Here's how the part is built. I have some questions about the finished solid (model axes, mm). Face numbers are marked on the shaded views. Coordinates: 2 decimals unless noted, no trailing zeros. Use one line per item in the form item = value. Start each with the question number.
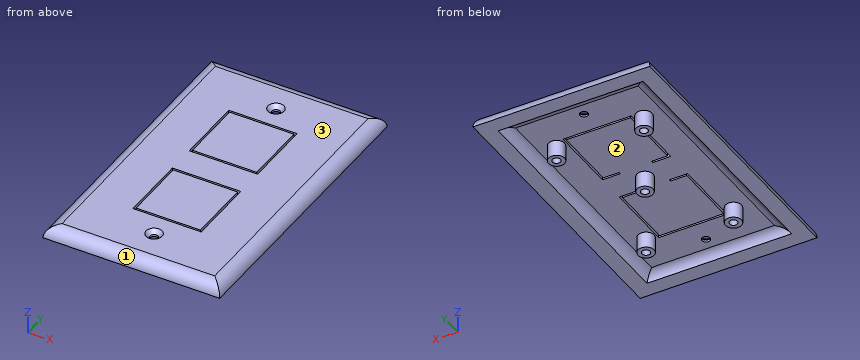
from build123d import *

# Parameters (mm, degrees)
F0_W        = 69.85
F0_H        = 114.3
F0_R        = 1.5875
F1_DEPTH    = 4.7625
F2_R        = 4.76249
F3_SIZE     = 1.5875
F4_W        = 57.15
F4_H        = 101.6
F5_DEPTH    = 2.38125
F6_T1_DEPTH = 101.6
F6_T3_DEPTH = 57.15
F8_DEPTH    = 4.7635
F7_W        = 12.7
F7_H        = 0.79375
F9_DEPTH    = 1.5875
F10_R       = 3.175
F10_R_2     = 1.5875
F11_DEPTH   = 6.35


# Not quite as in the source:
# - a fillet or chamfer that OpenCascade refuses, or shapes differently, is made with other operations: its cross-section is extruded or revolved along the edge and cut away or added
# - a fillet or chamfer is up to 0.001 mm smaller than in the source, because OpenCascade refuses the exact size


with BuildPart() as f1:
    # F0 (on Top) → F1 (new body)
    with BuildSketch(Plane.XY):
        Rectangle(F0_W, F0_H)
        with Locations((0, -41.6687)):
            Circle(F0_R, mode=Mode.SUBTRACT)
        with Locations((0, 41.6687)):
            Circle(F0_R, mode=Mode.SUBTRACT)
    extrude(amount=F1_DEPTH)

    # F2 (radius 4.7625 in the source; OpenCascade refuses exactly that, so slightly less here)
    f2_edges = [f1.edges().sort_by_distance(p)[0] for p in [
        (34.925, 0, 4.7625),
        (0, -57.15, 4.7625),
        (-34.925, 0, 4.7625),
        (0, 57.15, 4.7625),
    ]]
    fillet(f2_edges, radius=F2_R)

    # F3
    f3_edges = [f1.edges().sort_by_distance(p)[0] for p in [
        (-1.5875, 41.6687, 4.7625),
        (-1.5875, -41.6687, 4.7625),
    ]]
    chamfer(f3_edges, length=F3_SIZE)

    # F4 (on face) → F5 (cut)
    with BuildSketch(Plane(origin=(0, 0, 0), x_dir=(1, 0, 0), z_dir=(0, 0, -1))):
        Rectangle(F4_W, F4_H)
    extrude(amount=-F5_DEPTH, mode=Mode.SUBTRACT)

    # F6: fillet of radius 5.08 on 4 edges, made by hand

    # F6_s2 → F6_t1 (join)
    with BuildSketch(Plane.XZ.offset(-50.8)):
        with BuildLine():
            ThreePointArc((24.2711472565, 2.38125), (26.7304916814, 1.74625), (28.575, 0))
            Line((28.575, 0), (28.575, 2.38125))
            Line((28.575, 2.38125), (24.2711472565, 2.38125))
        make_face()
        with BuildLine():
            ThreePointArc((-24.2711472565, 2.38125), (-26.7304916814, 1.74625), (-28.575, 0))
            Line((-28.575, 0), (-28.575, 2.38125))
            Line((-28.575, 2.38125), (-24.2711472565, 2.38125))
        make_face()
    extrude(amount=F6_T1_DEPTH)

    # F6_s4 → F6_t3 (join)
    with BuildSketch(Plane.YZ.offset(-28.575)):
        with BuildLine():
            ThreePointArc((-46.4961472565, 2.38125), (-48.9554916814, 1.74625), (-50.8, 0))
            Line((-50.8, 0), (-50.8, 2.38125))
            Line((-50.8, 2.38125), (-46.4961472565, 2.38125))
        make_face()
        with BuildLine():
            ThreePointArc((46.4961472565, 2.38125), (48.9554916814, 1.74625), (50.8, 0))
            Line((50.8, 0), (50.8, 2.38125))
            Line((50.8, 2.38125), (46.4961472565, 2.38125))
        make_face()
    extrude(amount=F6_T3_DEPTH)

    # F7 (on face) → F8 (cut, through all)
    with BuildSketch(Plane.XY.offset(4.7625)):
        Polygon((-12.7, 31.94685), (12.7, 31.94685), (12.7, 6.54685), (6.35, 6.54685), (6.35, 5.7531), (13.49375, 5.7531), (13.49375, 32.7406), (-13.49375, 32.7406), (-13.49375, 5.7531), (-6.35, 5.7531), (-6.35, 6.54685), (-12.7, 6.54685), align=None)
        Polygon((6.35, -5.7531), (6.35, -6.54685), (12.7, -6.54685), (12.7, -31.94685), (-12.7, -31.94685), (-12.7, -6.54685), (-6.35, -6.54685), (-6.35, -5.7531), (-13.49375, -5.7531), (-13.49375, -32.7406), (13.49375, -32.7406), (13.49375, -5.7531), align=None)
    extrude(amount=-F8_DEPTH, mode=Mode.SUBTRACT)

    # F7 (on face) → F9 (cut)
    with BuildSketch(Plane.XY.offset(4.7625)):
        with Locations((0, 6.149975)):
            Rectangle(F7_W, F7_H)
        with Locations((0, -6.149975)):
            Rectangle(F7_W, F7_H)
    extrude(amount=-F9_DEPTH, mode=Mode.SUBTRACT)

    # F10 (on face) → F11 (join)
    with BuildSketch(Plane(origin=(0, 0, 2.38125), x_dir=(1, 0, 0), z_dir=(0, 0, -1))):
        with Locations((-17.272, 30.6211472565)):
            Circle(F10_R)
        with Locations((-17.272, 30.6211472565)):
            Circle(F10_R_2, mode=Mode.SUBTRACT)
        with Locations((-17.272, -30.5562)):
            Circle(F10_R)
        with Locations((-17.272, -30.6211472565)):
            Circle(F10_R_2, mode=Mode.SUBTRACT)
        with Locations((17.272, 30.6211472565)):
            Circle(F10_R)
        with Locations((17.272, 30.6211472565)):
            Circle(F10_R_2, mode=Mode.SUBTRACT)
        with Locations((17.272, -30.5562)):
            Circle(F10_R)
        with Locations((17.272, -30.6211472565)):
            Circle(F10_R_2, mode=Mode.SUBTRACT)
        Circle(F10_R)
        Circle(F10_R_2, mode=Mode.SUBTRACT)
    extrude(amount=F11_DEPTH)


solid = f1.part
1) If we mould it in two halves opening along Y, with no side actions, what happens to the marked faces 1, 2 and 3? For each: pulls with the +Y half, pulls with the -Y half, needs draft (parallel to the pull), parting line crosses it, or undercut.
2) Suppose I cut it at A-A, the plane y = 21.5. Give the number of separate pieces and of enclosed holes in the cut face, then the cut area to 3 significant figures.
3) I need wall thicknesses on probe 1 along X at (y, z) = (30.5, -1.75); probe 2 along X at (y, z) = (-32, 1); probe 3 along X at (y, z) = (0.5, 1.25). Which ranges of each line are inside material? Lowest first, please. Write a range as [from, to].
4) For pin 1 (0.6 mm diameter, centred on y = -6, z = 2.5, fed in from -X); pin 2 (0.7 mm diameter, centred on x = -2.5, z = 3.5, fed in from +Y); pin 3 (1.2 mm diameter, centred on x = 5, z = 3.5, fed in from +Y), each with a flat end and sliding along its axis, tell me the tip position at first contact or that it passes through.
From the geometry:
q1.face_1 = pulls with the -Y half
q1.face_2 = undercut
q1.face_3 = needs draft
q2.separate_pieces = 3
q2.enclosed_holes = 0
q2.area = 189 mm2
q3.probe_1 = [-20.45, -18.85], [-15.69, -14.1], [14.1, 15.69], [18.85, 20.45]
q3.probe_2 = [-34.82, -27.75], [-20.13, -18.06], [-16.49, -14.41], [14.41, 16.49], [18.06, 20.13], [27.75, 34.82]
q3.probe_3 = [-34.76, -27.47], [-3.14, -1.51], [1.51, 3.14], [27.47, 34.76]
q4.pin_1 = -34.39
q4.pin_2 = 55.96
q4.pin_3 = 56.17
